Geometry: final body of the model. Coordinates: model frame, mm. A direction names the side the tool comes from. Give positions to 0.01 mm unless a question says otherwise; leave off trailing zeros. Write each loop counter-clockwise with the first axis right and the second up, starting at its lowest first coordinate (ties: lowest second). Pieces come first, ordered by that corner, then holes.
Q1. Section C-C (z = -1.3). Return the cut outline in (x, y), plus the area to 3 significant figures.
Q2. Line query: line 1 (Z direction, x = 17, y = -2); line 2 (Y direction, x = 0.5, z = -1.45); line 3 (X direction, y = -2, z = 0.9). Output: solid intervals per line, ascending.
Q3. Reachability of faces 1 (the cylindrical face through (-1.71, 0.72, 0.59)), 2 (the flat face through (-4, 0, 1.7)) from +Z, -Z, +X, -X, +Y, -Y: full face, straight path, thin tool, end or side. Return the list, or none.
Q4. Section A-A (x = 0). Return the cut outline in (y, z), plus the area to 3 significant figures.
Q5. Section B-B (y = 0). Return the cut outline in (x, z).
Q6. Mould query, pull axis X, two halves, no side actions, for faces 3 (the flat face through (0, 0, -2)), 4 (the cylindrical face through (-4.336, -19.524, -1.24)), 5 (the cylindrical face through (6.217, -0.919, 0.592)). Classes: +X half, -X half, draft (parallel to the pull), parting line (faces both ways), or undercut.
Q7. Pin query (flat end, axial travel): pin 1 Ø12 at (x, y) = (-12.5, 8.5) entering from +Z; pin 2 Ø1.5 at (x, z) = (-7.5, 0) entering from -Y; pin 3 Ø19.5 at (x, y) = (-2.5, 7.5) entering from +Z. Return the tip coordinate at first contact, or that it passes through.
from build123d import *

# Parameters (mm, degrees)
F0_R     = 2.4
F1_DEPTH = 1.7
F0_R_2   = 20
F2_DEPTH = 2
F3_R     = 0.5
F4_DEPTH = 2


with BuildPart() as f1:
    # F0 (on Top) → F1 (new body)
    with BuildSketch(Plane.XY):
        with Locations((-4, 0)):
            Circle(F0_R)
    extrude(amount=F1_DEPTH)



with BuildPart() as f1b:
    # F0 (on Top) → F1, piece 2 (new body)
    with BuildSketch(Plane.XY):
        with Locations((4, 0)):
            Circle(F0_R)
    extrude(amount=F1_DEPTH)


with BuildPart() as f1_1:
    add(f1.part)

    add(f1b.part)  # F2 merges F1b
    # F0 (on Top) → F2 (join)
    with BuildSketch(Plane.XY):
        Circle(F0_R_2)
        with Locations((-4, 0)):
            Circle(F0_R, mode=Mode.SUBTRACT)
        with Locations((4, 0)):
            Circle(F0_R, mode=Mode.SUBTRACT)
    extrude(amount=-F2_DEPTH)

    # F3
    f3_edges = [f1_1.edges().sort_by_distance(p)[0] for p in [
        (-6.4, 0, 1.7),
        (1.6, 0, 1.7),
        (-20, 0, 0),
    ]]
    fillet(f3_edges, radius=F3_R)

    # F4 (add): faces of the model
    f4_faces = [f1_1.faces().sort_by_distance(p)[0] for p in [
        (-4, 0, 0),
        (4, 0, 0),
    ]]
    extrude(f4_faces, amount=F4_DEPTH)


solid = f1_1.part
Computed:
1. outline: circle Ø40 at (0, 0)
1. area: 1,260 mm2
2. line 1: z = -2 to 0
2. line 2: y = -19.99 to 19.99
2. line 3: x = -5.33 to -2.67, 2.67 to 5.33
3. face 1: +Z
3. face 2: +Z, +X, -X, +Y, -Y
4. outline: (-20, -2) - (20, -2) - (20, -0.5) arc R0.5 ccw to (19.5, 0) - (-19.5, 0) arc R0.5 ccw to (-20, -0.5) - close
4. area: 79.9 mm2
5. outline: (-20, -2) - (20, -2) - (20, -0.5) arc R0.5 ccw to (19.5, 0) - (6.4, 0) - (6.4, 1.2) arc R0.5 ccw to (5.9, 1.7) - (2.1, 1.7) arc R0.5 ccw to (1.6, 1.2) - (1.6, 0) - (-1.6, 0) - (-1.6, 1.2) arc R0.5 ccw to (-2.1, 1.7) - (-5.9, 1.7) arc R0.5 ccw to (-6.4, 1.2) - (-6.4, 0) - (-19.5, 0) arc R0.5 ccw to (-20, -0.5) - close
6. face 3: draft
6. face 4: parting line
6. face 5: undercut
7. pin 1: stops at z = 0
7. pin 2: stops at y = -18.77
7. pin 3: stops at z = 1.7
